Geometry check sheet. Reference: the model listing, model coordinates, mm. Face numbers are marked on the shaded views. A direction names the side the tool comes from. Coordinates: 2 decimals unless noted, no trailing zeros. Write each loop counter-clockwise with the first axis right and the second up, starting at its lowest first coordinate (ties: lowest second). Pieces come first, ordered by that corner, then holes. Notation, with made-up numbers: (49.25, -15.5) -> (94.25, -15.5) arc R7 ccw to (94.25, -8.5) -> close; hole circle Ø9 at (-30, -23.5). An arc over 180 degrees is marked (long way). Answer in a Markdown table with one row per item. Add a question column.
1. Cross-section at B-B on x = 38. Record the cut outline in (y, z), and give its area (3 significant figures).
2. Scan lines: L1, parallel to Z at x = 10.5, y = 0.25; L2, parallel to X at y = -2.5, z = 1.5; L3, parallel to X at y = 3.5, z = -1.5. Record each from-to range of solid material in increasing order. Write a range as from..to.
3. Depth check by flat-ended pin: P1, Ø4, axis at x = 60.5, z = 3, coming from the +Y side; P2, Ø1.5, axis at x = 44, y = 3, coming from the +Z side; P3, Ø5, axis at x = 50, z = -2, coming from the +Y side; P4, Ø1, axis at x = 5, z = 4, coming from the -Y side. Enter the tip coordinate at first touch or a pass-through.
4. Set-up check for the marked faces 1 and 2: record each of +Z, -Z, +X, -X, +Y, -Y from which the full face is reachable in a straight line by a thin tool's end or side.
5. Cross-section at A-A on y = 0. Record the cut outline in (x, z).
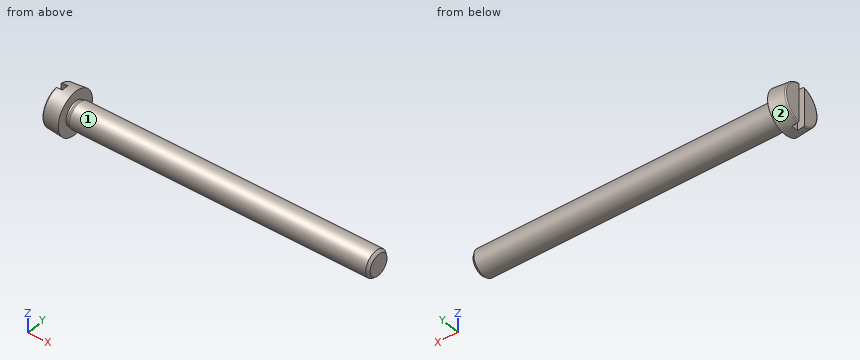
Autodesk Inventor part; units mm, degrees
ref_plane "Work Plane1" through (30.1625, 0, 0) normal (0, 0, -1) x (1, 0, 0)
ref_plane "YZ Plane" through (0, 0, 0) normal (1, 0, 0) x (0, 1, 0)
ref_plane "XZ Plane" through (0, 0, 0) normal (0, 1, 0) x (-1, 0, 0)
sketch "Skizze1" plane through (0, 0, 0) normal (0, 0, 1) x (1, 0, 0)
  line L0 (-3.9, 0) -> (70, 0)
  line L1 (70, 0) -> (70, 3)
  line L2 (70, 3) -> (1, 3)
  line L3 (1, 3) -> (0.3864, 2.7294)
  line L4 (0.3864, 2.7294) -> (0, 2.7294)
  line L5 (0, 2.7294) -> (0, 5)
  line L6 (-18.68, 0) -> (84.78, 0)
  line L7 (0, -1) -> (0, 6)
  line L8 (-3.9, 0) -> (-3.9, 4.6588)
  line L9 (0, 5) -> (-3.9, 4.6588)
  line L10 (1, 3) -> (0, 3) construction
  dimension "d0" = 70
  dimension "d1" = 69
  dimension "d2" = 0.6136
  dimension "d3" = 3.9
  dimension "d4" = 6
  dimension "d5" = 5.4587
  dimension "d9" = 10
  dimension "d10" = 5
revolve "Körper" add sketch "Skizze1" angle 360 about axis through (-3.9, 0, 0) along (1, 0, 0)
sketch "Skizze2" plane through (-3.9, 0, 0) normal (-1, 0, 0) x (0, 0, 1)
  circle A0 centre (0, 0) radius 5
  line L0 (0, 0) -> (0, 4.6588)
  line L1 (-5, 0.8) -> (5, 0.8)
  line L2 (5, 0.8) -> (5, -0.8)
  line L3 (5, -0.8) -> (-5, -0.8)
  line L4 (-5, -0.8) -> (-5, 0.8)
  line L5 (-5, 0) -> (5, 0) construction
  line L6 (0, 0.8) -> (0, -0.8) construction
  dimension "d11" = 1.6
  dimension "d12" = 10
fillet "Rundung1" radius 0.25 1 edges at (-3.9, -4.6588, 0)
extrude "Loch" cut sketch "Skizze2" against normal blind 1.6 contours A0 L3 L1 | L2 L3 A0 | A0 L1 L2 | A0 L4 L1 | L3 L4 A0
thread "Gewinde"
chamfer "Fase1" distance 0.5413 distance2 0.6136 1 edges at (70, -3, 0) measured on face at (70, 1.3648, -1.3588)
ref_plane "Work Plane1" through (30.1625, 0, 0) normal (0, 0, -1) x (1, 0, 0)
equation "\"d11\" = SBR"
equation "\"d12\" = KOD"
equation "\"d14\" = RR"
equation "\"d19\" = STI"
equation "\"d15\" = GEL"
equation "\"d17\" = -0.5 * SPD + 0.5 * GD"
equation "\"d3\" = KOH"
equation "\"d4\" = GD"
equation "\"d5\" = BDM"
equation "\"d9\" = KOD"
equation "\"d10\" = KEWI"
equation "\"GD\" = 6"
equation "\"GEL\" = 38"
equation "\"KOD\" = 10"
equation "\"KOH\" = 3.9"
equation "\"GAL\" = 0.61345 * PTC"
equation "\"SPD\" = 4.91747"
equation "\"BDM\" = 5.45873"
equation "\"GUL\" = 0.61345 * PTC"
equation "\"RR\" = 0.25"
equation "\"SBR\" = 1.6"
equation "\"STI\" = 1.6"
equation "\"KEWI\" = 5deg"
equation "\"PTC\" = 1"
equation "\"THREADDIA\" = 6"
equation "\"TOA\" = 30deg"
equation "\"NND\" = 6"
equation "\"GD1\" = THREADDIA - 1.2269 * PTC"
properties part number "DIN 84 - M6 x 70" material "Stahl, weich"
Results found:
| question | item | result |
|---|---|---|
| 1 | outline | circle Ø6 at (0, 0) |
| 1 | area | 28.3 mm^2 |
| 2 | L1 | z = -2.99..2.99 |
| 2 | L2 | x = -3.9..0, 0.81..69.48 |
| 2 | L3 | x = -3.9..0 |
| 3 | P1 | stops at y = 2.83 |
| 3 | P2 | stops at z = 1.98 |
| 3 | P3 | stops at y = 3 |
| 3 | P4 | passes through |
| 4 | face 1 | +X |
| 4 | face 2 | -X |
| 5 | outline | (-2.3, -4.8) -> (0, -5) -> (0, -2.73) -> (0.39, -2.73) -> (1, -3) -> (69.39, -3) -> (70, -2.46) -> (70, 2.46) -> (69.39, 3) -> (1, 3) -> (0.39, 2.73) -> (0, 2.73) -> (0, 5) -> (-2.3, 4.8) -> close |
